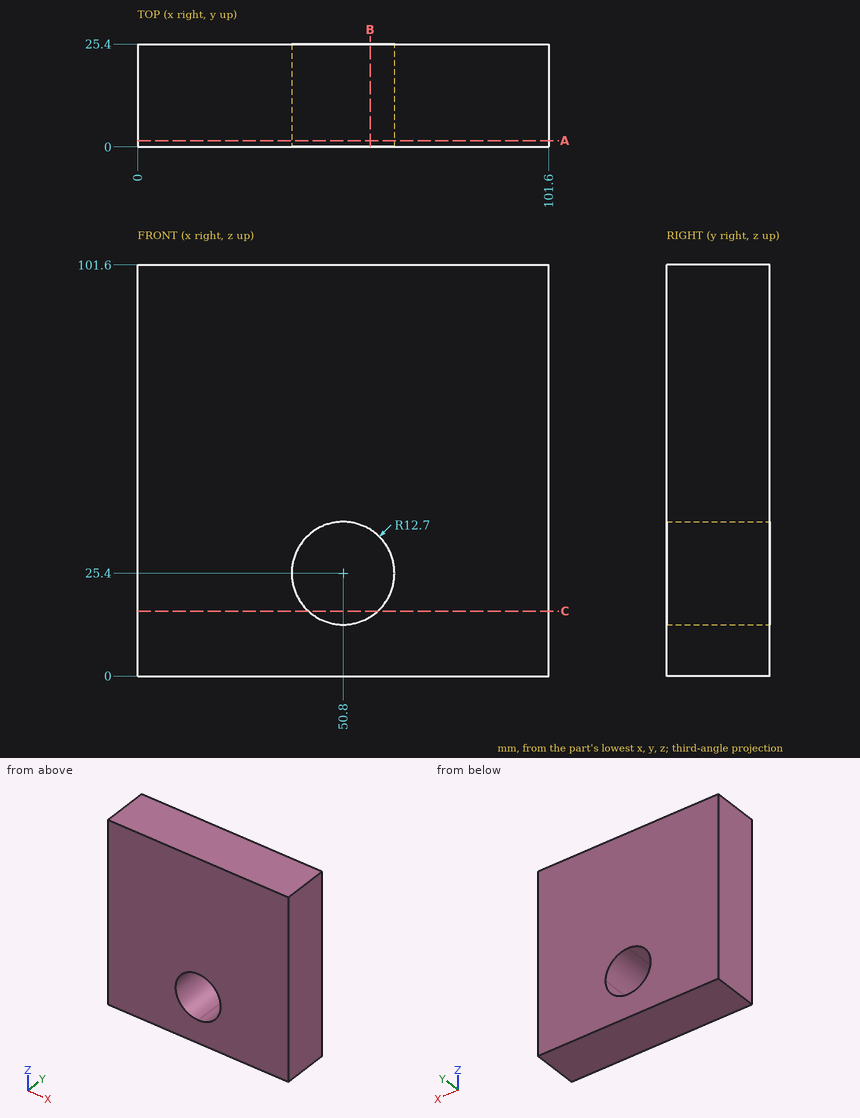
Design review of the part shown in the three views and the two pictorial views. Dimensions are in mm from the part's minimum x, y and z. Round coordinates to 2 decimals unless told otherwise and drop trailing zeros. Order: outer loops, then holes, each group sorted by start corner. A loop starts at its lowest first (then second) coordinate and runs counter-clockwise, first axis right, second up.
(1) Wall thickness on L1, parallel to Z at x = 50.5, y = 7.25; L2, parallel to X at y = 20.75, z = 23; L3, parallel to X at y = 1.5, z = 31: over which ranges is each line inside the solid? List them lowest first.
Working result:
L1: z = 0 to 12.7, 38.1 to 101.6
L2: x = 0 to 38.33, 63.27 to 101.6
L3: x = 0 to 39.4, 62.2 to 101.6
(2) Take a section at C-C, the plane z = 16. State the section outline as (x, y) points.
Working result:
outline: (0, 0) - (42.26, 0) - (42.26, 25.4) - (0, 25.4) - close; (59.34, 0) - (101.6, 0) - (101.6, 25.4) - (59.34, 25.4) - close
(3) Take a section at B-B, the plane x = 57.5. State the section outline as (y, z) points.
Working result:
outline: (0, 0) - (25.4, 0) - (25.4, 14.61) - (0, 14.61) - close; (0, 36.19) - (25.4, 36.19) - (25.4, 101.6) - (0, 101.6) - close
(4) Take a section at A-A, the plane y = 1.5. State the section outline as (x, z) points, plus the area to 3 significant figures.
Working result:
outline: (0, 0) - (101.6, 0) - (101.6, 101.6) - (0, 101.6) - close; hole circle Ø25.4 at (50.8, 25.4)
area: 9,820 mm2
